```python
from build123d import *

# Parameters (mm, degrees)
BOSS_EXTRUDE2_DEPTH = 101.6


with BuildPart() as part:
    # Sketch1 → Boss-Extrude2 (new body)
    with BuildSketch(Plane.XY):
        with BuildLine():
            Line((-30.375497444, 98.732937893), (-11.325497444, 98.732937893))
            Line((-11.325497444, 98.732937893), (-11.325497444, 121.592937893))
            ThreePointArc((-11.325497444, 121.592937893), (-10.581548668, 123.388989117), (-8.785497444, 124.132937893))
            Line((-8.785497444, 124.132937893), (8.785497444, 124.132937893))
            ThreePointArc((8.785497444, 124.132937893), (10.581548668, 123.388989117), (11.325497444, 121.592937893))
            Line((11.325497444, 121.592937893), (11.325497444, 98.732937893))
            Line((11.325497444, 98.732937893), (30.375497444, 98.732937893))
            Line((30.375497444, 98.732937893), (30.375497444, 73.332937893))
            ThreePointArc((30.375497444, 73.332937893), (0, 79.375), (-30.375497444, 73.332937893))
            Line((-30.375497444, 73.332937893), (-30.375497444, 98.732937893))
        make_face()
    extrude(amount=BOSS_EXTRUDE2_DEPTH)


solid = part.part
```
Design review of the part built by this model. Coordinates are the model's own, in mm. A direction names the side the tool comes from. Give positions to 0.01 mm unless a question says otherwise; leave off trailing zeros. Order: outer loops, then holes, each group sorted by start corner. A loop starts at its lowest first (then second) coordinate and runs counter-clockwise, first axis right, second up. Notation, with made-up numbers: M 65,43.5 L 104,43.5 A27 ccw 104,79.5 Z; hole C 4.25,72.25 d2. An arc over 180 degrees is marked long. One line per question, with ' | ' between items. Start each with the question number.
Q1. For pin 1 Ø2 at (x, z) = (-5, 76.5) entering from -Y; pin 2 Ø10 at (y, z) = (113, 29) entering from +X; pin 3 Ø15 at (x, z) = (-23, 33.5) entering from +Y, all flat-tipped, find the tip position at first contact; note any pin that passes through.
Q2. Machinability: for faces 1 (the face through (11.325, 110, 50)), 2 (the face through (-21, 98.733, 50)), 3 (the face through (0, 124.133, 50)), which of the approach directions +Z, -Z, +X, -X, +Y, -Y give a long, thin tool a straight path to every point of the face, cutting with its end or side? Answer none if there is none.
Q3. For L1, parallel to X at y = 119, z = 16; L2, parallel to Y at x = -7, z = 51; L3, parallel to Y at x = -25, z = 82, list the stretches that pass through material, from the lowest coordinate up. Write a range as [from, to].
Q4. We need section B-B (y = 76). Write out the cut boundary in (x, z), plus the area to 3 significant figures.
Q5. We need section D-D (x = -21). Write out the cut boundary in (y, z).
Q6. The part is to be moulded in two halves that separate along X. For faces 4 (the face through (0.436, 79.374, 50.089)), 5 (the face through (30.375, 86, 50)), 6 (the face through (-11.325, 110, 50)), 7 (the face through (21, 98.733, 50)), say which applies: +X half, -X half, draft (parallel to the pull), parting line (faces both ways), or undercut.
Q7. We need section C-C (y = 110.5). Write out the cut boundary in (x, z), plus the area to 3 significant figures.
Returned:
1) pin 1: y = 79.15 | pin 2: x = 11.33 | pin 3: y = 98.73
2) face 1: +Z, -Z, +X, +Y | face 2: +Z, -Z, -X, +Y | face 3: +Z, -Z, +X, -X, +Y
3) L1: [-11.33, 11.33] | L2: [79.07, 124.13] | L3: [75.34, 98.73]
4) outline: M -30.38,0 L -22.9,0 L -22.9,101.6 L -30.38,101.6 Z; M 22.9,0 L 30.38,0 L 30.38,101.6 L 22.9,101.6 Z | area: 1,520 mm2
5) outline: M 76.55,0 L 98.73,0 L 98.73,101.6 L 76.55,101.6 Z
6) face 4: undercut | face 5: +X half | face 6: -X half | face 7: draft
7) outline: M -11.33,0 L 11.33,0 L 11.33,101.6 L -11.33,101.6 Z | area: 2,300 mm2
